Autodesk Inventor part; units mm, degrees
ref_plane "YZ Plane" through (0, 0, 0) normal (1, 0, 0) x (0, 1, 0)
ref_plane "XZ Plane" through (0, 0, 0) normal (0, 1, 0) x (-1, 0, 0)
ref_plane "XY Plane" through (0, 0, 0) normal (0, 0, 1) x (1, 0, 0)
sketch "Sketch1" plane through (0, 0, 0) normal (0, 0, 1) x (1, 0, 0)
  line L0 (49.1624, -46.1074) -> (-32.1176, -46.1074)
  line L1 (49.1624, 19.9326) -> (49.1624, -46.1074)
  line L2 (49.1624, -46.1074) -> (49.1624, 19.9326)
  line L3 (-32.1176, 19.9326) -> (49.1624, 19.9326)
  line L4 (49.1624, 19.9326) -> (-32.1176, 19.9326)
  line L5 (-32.1176, -46.1074) -> (-32.1176, 19.9326)
  line L6 (-32.1176, 19.9326) -> (-32.1176, -46.1074)
  line L7 (-32.1176, -46.1074) -> (49.1624, -46.1074)
  line L8 (47.5774, -44.8414) -> (38.8489, -44.8414)
  line L9 (47.5774, -44.8414) -> (38.8489, -44.8414)
  line L10 (38.8489, -40.9552) -> (38.8489, -44.8414)
  line L11 (38.8489, -44.8414) -> (38.8489, -40.9552)
  line L12 (38.8489, -40.9552) -> (47.5774, -40.9552)
  line L13 (38.8489, -40.9552) -> (47.5774, -40.9552)
  line L14 (47.5774, -40.9552) -> (47.5774, -44.8414)
  line L15 (47.5774, -40.9552) -> (47.5774, -44.8414)
  line L16 (47.5774, 14.7804) -> (38.8489, 14.7804)
  line L17 (47.5774, 14.7804) -> (38.8489, 14.7804)
  line L18 (38.8489, 14.7804) -> (38.8489, 18.6666)
  line L19 (38.8489, 14.7804) -> (38.8489, 18.6666)
  line L20 (38.8489, 18.6666) -> (47.5774, 18.6666)
  line L21 (38.8489, 18.6666) -> (47.5774, 18.6666)
  line L22 (47.5774, 18.6666) -> (47.5774, 14.7804)
  line L23 (47.5774, 18.6666) -> (47.5774, 14.7804)
  line L24 (31.2541, -44.8414) -> (21.8023, -44.8414)
  line L25 (31.2541, -44.8414) -> (21.8023, -44.8414)
  line L26 (21.8023, -40.9552) -> (21.8023, -44.8414)
  line L27 (21.8023, -44.8414) -> (21.8023, -40.9552)
  line L28 (21.8023, -40.9552) -> (31.2541, -40.9552)
  line L29 (31.2541, -40.9552) -> (31.2541, -44.8414)
  line L30 (31.2541, -40.9552) -> (31.2541, -44.8414)
  line L31 (-4.7575, -44.8414) -> (-14.2093, -44.8414)
  line L32 (-4.7575, -44.8414) -> (-14.2093, -44.8414)
  line L33 (-14.2093, -40.9552) -> (-14.2093, -44.8414)
  line L34 (-14.2093, -44.8414) -> (-14.2093, -40.9552)
  line L35 (-4.7575, -40.9552) -> (-14.2093, -40.9552)
  line L36 (-14.2093, -40.9552) -> (-4.7575, -40.9552)
  line L37 (-4.7575, -40.9552) -> (-4.7575, -44.8414)
  line L38 (-4.7575, -40.9552) -> (-4.7575, -44.8414)
  line L39 (-21.804, -40.9552) -> (-21.804, -44.8414)
  line L40 (-30.5326, -44.8414) -> (-21.804, -44.8414)
  line L41 (-21.804, -44.8414) -> (-30.5326, -44.8414)
  line L42 (-30.5326, -44.8414) -> (-30.5326, -40.9552)
  line L43 (-30.5326, -40.9552) -> (-21.804, -40.9552)
  line L44 (-30.5326, -40.9552) -> (-21.804, -40.9552)
  line L45 (-21.804, -40.9552) -> (-21.804, -44.8414)
  line L46 (31.2541, 14.7804) -> (21.8023, 14.7804)
  line L47 (31.2541, 14.7804) -> (21.8023, 14.7804)
  line L48 (21.8023, 14.7804) -> (21.8023, 18.6666)
  line L49 (21.8023, 14.7804) -> (21.8023, 18.6666)
  line L50 (21.8023, 18.6666) -> (31.2541, 18.6666)
  line L51 (21.8023, 18.6666) -> (31.2541, 18.6666)
  line L52 (31.2541, 18.6666) -> (31.2541, 14.7804)
  line L53 (31.2541, 18.6666) -> (31.2541, 14.7804)
  line L54 (3.2185, 14.7804) -> (13.8264, 14.7804)
  line L55 (13.8264, 14.7804) -> (3.2185, 14.7804)
  line L56 (3.2185, 18.6666) -> (3.2185, 14.7804)
  line L57 (3.2185, 14.7804) -> (3.2185, 18.6666)
  line L58 (3.2185, 18.6666) -> (13.8264, 18.6666)
  line L59 (3.2185, 18.6666) -> (13.8264, 18.6666)
  line L60 (13.8264, 14.7804) -> (13.8264, 18.6666)
  line L61 (13.8264, 18.6666) -> (13.8264, 14.7804)
  line L62 (-4.7575, 14.7804) -> (-14.2093, 14.7804)
  line L63 (-4.7575, 14.7804) -> (-14.2093, 14.7804)
  line L64 (-14.2093, 14.7804) -> (-14.2093, 18.6666)
  line L65 (-14.2093, 14.7804) -> (-14.2093, 18.6666)
  line L66 (-14.2093, 18.6666) -> (-4.7575, 18.6666)
  line L67 (-14.2093, 18.6666) -> (-4.7575, 18.6666)
  line L68 (-4.7575, 18.6666) -> (-4.7575, 14.7804)
  line L69 (-4.7575, 18.6666) -> (-4.7575, 14.7804)
  line L70 (-21.804, 18.6666) -> (-21.804, 14.7804)
  line L71 (-21.804, 14.7804) -> (-30.5326, 14.7804)
  line L72 (-21.804, 14.7804) -> (-30.5326, 14.7804)
  line L73 (-30.5326, 18.6666) -> (-21.804, 18.6666)
  line L74 (-30.5326, 14.7804) -> (-30.5326, 18.6666)
  line L75 (-30.5326, 18.6666) -> (-21.804, 18.6666)
  line L76 (-21.804, 18.6666) -> (-21.804, 14.7804)
  point P0 (0, 0)
  point P1 (0, 0)
extrude "Extrusion1" add sketch "Sketch1" along normal blind 2.286
sketch "Sketch2" plane through (0, 0, 2.286) normal (0, 0, 1) x (1, 0, 0)
  line L0 (-30.5326, 18.6666) -> (-30.5326, 14.7804)
  line L1 (47.5774, 18.6666) -> (38.8489, 18.6666)
  line L2 (-30.5326, 18.6666) -> (47.5774, 18.6666)
  line L3 (47.5774, 18.6666) -> (47.5774, 14.7804)
  line L4 (47.5774, 18.6666) -> (47.5774, 14.7804)
  line L5 (-30.5326, 14.7804) -> (-21.804, 14.7804)
  line L6 (47.5774, 14.7804) -> (-30.5326, 14.7804)
  line L7 (-21.804, 18.6666) -> (-21.804, 14.7804)
  line L8 (-21.804, 18.6666) -> (-21.804, 14.7804)
  line L9 (-4.7575, 18.6666) -> (-14.2093, 18.6666)
  line L10 (-14.2093, 14.7804) -> (-14.2093, 18.6666)
  line L11 (-14.2093, 18.6666) -> (-14.2093, 14.7804)
  line L12 (3.2185, 14.7804) -> (3.2185, 18.6666)
  line L13 (3.2185, 18.6666) -> (3.2185, 14.7804)
  line L14 (13.8264, 18.6666) -> (13.8264, 14.7804)
  line L15 (13.8264, 18.6666) -> (13.8264, 14.7804)
  line L16 (21.8023, 18.6666) -> (21.8023, 14.7804)
  line L17 (31.2541, 18.6666) -> (31.2541, 14.7804)
  line L18 (31.2541, 18.6666) -> (31.2541, 14.7804)
  line L19 (38.8489, 14.7804) -> (47.5774, 14.7804)
  line L20 (38.8489, 18.6666) -> (38.8489, 14.7804)
  point P0 (0, 0)
properties part number "mcdave_scelevel"
Here's how the part is built. I have some questions about the finished solid (model axes, mm). Coordinates: 2 decimals unless noted, no trailing zeros. Loops run counter-clockwise (first coordinate to the right, second up) from the corner with the lowest first, then second, coordinate; pieces in that order, holes last. Notation, with made-up numbers: M -37,-14 L -7,-14 A11 ccw -7,-6 Z; hole C -14,21.25 d4. An arc over 180 degrees is marked long. One line per item, written item: value.
1. Imagine slicing it at A-A (x = 10). List the corners of the cut face in (y, z) for me.
Geometry says:
outline: M -46.11,0 L 14.78,0 L 14.78,2.29 L -46.11,2.29 Z; M 18.67,0 L 19.93,0 L 19.93,2.29 L 18.67,2.29 Z
2. Imagine slicing it at B-B (x = 26). List the corners of the cut face in (y, z) for me, and give its area (3 significant figures).
Geometry says:
outline: M -46.11,0 L -44.84,0 L -44.84,2.29 L -46.11,2.29 Z; M -40.96,0 L 14.78,0 L 14.78,2.29 L -40.96,2.29 Z; M 18.67,0 L 19.93,0 L 19.93,2.29 L 18.67,2.29 Z
area: 133 mm2
3. Imagine slicing it at C-C (z = 0.5). State how many separate pieces and enclosed holes the cut face has, and give its area (3 significant figures).
Geometry says:
separate pieces: 1
enclosed holes: 9
area: 5,040 mm2
4. Will this pin go through, and if not, where does the flat tip stop? pin 1 Ø2 at (x, y) = (23.5, -12.5) entering from -Z.
Geometry says:
pin 1: stops at z = 0
5. Please list where these lines run through material, in increasing order: probe 1 along Y at (x, z) = (-28, 0.1); probe 2 along Y at (x, z) = (13.5, 1.2).
Geometry says:
probe 1: y = -46.11 to -44.84, -40.96 to 14.78, 18.67 to 19.93
probe 2: y = -46.11 to 14.78, 18.67 to 19.93
6. Thinking about a two-plate mould opening in Y: for faces 1 (the flat face through (-9, -44.841, 1)), 2 (the flat face through (43, 14.78, 1)), 3 (the flat face through (49.162, -13, 1)), which applies, +Y half, -Y half, draft (parallel to the pull), parting line (faces both ways), or undercut?
Geometry says:
face 1: undercut
face 2: undercut
face 3: draft
